```python
from build123d import *

# Parameters (mm, degrees)
CROQUIS1_R              = 1
SALIENTE_EXTRUIR1_DEPTH = 4
CROQUIS1_3_R            = 7
CROQUIS1_3_R_2          = 4
SALIENTE_EXTRUIR2_DEPTH = 6
CHAFL_N1_SIZE           = 3
CHAFL_N2_SIZE           = 3
CHAFL_N2_SIZE_2         = 0.803847577
SALIENTE_EXTRUIR3_DEPTH = 4
MATRIZC1_COUNT          = 36


with BuildPart() as part:
    # Croquis1 → Saliente-Extruir1 (new body)
    with BuildSketch(Plane(origin=(0, 0, 0), x_dir=(1, 0, 0), z_dir=(0, 1, 0))):
        with BuildLine():
            ThreePointArc((-7.395099729, 1.25), (0, -7.5), (7.395099729, 1.25))
            Line((7.395099729, 1.25), (2.958039892, 27.5))
            ThreePointArc((2.958039892, 27.5), (0, 30), (-2.958039892, 27.5))
            Line((-2.958039892, 27.5), (-7.395099729, 1.25))
        make_face()
        with Locations(Location((0, 24, 0), (0, 0, 270))):
            Circle(CROQUIS1_R, mode=Mode.SUBTRACT)
        with Locations(Location((0, 15, 0), (0, 0, 270))):
            Circle(CROQUIS1_R, mode=Mode.SUBTRACT)
        with Locations(Location((0, 18, 0), (0, 0, 270))):
            Circle(CROQUIS1_R, mode=Mode.SUBTRACT)
        with Locations(Location((0, 21, 0), (0, 0, 270))):
            Circle(CROQUIS1_R, mode=Mode.SUBTRACT)
        with Locations(Location((0, 27, 0), (0, 0, 270))):
            Circle(CROQUIS1_R, mode=Mode.SUBTRACT)
        with BuildLine():
            ThreePointArc((-2.988584094, 0.261467228), (-2.974334584, 0.391578577), (-2.954423259, 0.520944533))
            ThreePointArc((-2.954423259, 0.520944533), (2.974334584, -0.391578577), (-2.988584094, 0.261467228))
        make_face(mode=Mode.SUBTRACT)
    extrude(amount=SALIENTE_EXTRUIR1_DEPTH)

    # Croquis1<3> → Saliente-Extruir2 (add)
    # profile 1 of 3: a face of its own
    with BuildSketch(Plane(origin=(0, 0, 0), x_dir=(1, 0, 0), z_dir=(0, 1, 0))):
        with BuildLine():
            ThreePointArc((6.453329346, 3.82158872), (0, 7.5), (-6.453329346, 3.82158872))
            Line((-6.453329346, 3.82158872), (-6.90209308, 1.166666667))
            ThreePointArc((-6.90209308, 1.166666667), (0, 7), (6.90209308, 1.166666667))
            Line((6.90209308, 1.166666667), (6.453329346, 3.82158872))
        make_face()
    # profile 2 of 3: a face of its own
    with BuildSketch(Plane(origin=(0, 0, 0), x_dir=(1, 0, 0), z_dir=(0, 1, 0))):
        with BuildLine():
            Line((-5.662533507, 8.5), (-6.453329346, 3.82158872))
            ThreePointArc((-6.453329346, 3.82158872), (0, 7.5), (6.453329346, 3.82158872))
            Line((6.453329346, 3.82158872), (5.662533507, 8.5))
            Line((5.662533507, 8.5), (-5.662533507, 8.5))
        make_face()
    # profile 3 of 3: a face of its own
    with BuildSketch(Plane(origin=(0, 0, 0), x_dir=(1, 0, 0), z_dir=(0, 1, 0))):
        Circle(CROQUIS1_3_R)
        with Locations(Location((0, 0, 0), (0, 0, 270))):
            Circle(CROQUIS1_3_R_2, mode=Mode.SUBTRACT)
    extrude(amount=SALIENTE_EXTRUIR2_DEPTH)

    # Chaflán1
    # the kernel refuses this chamfer: 3 mm, written as the material it adds along each edge
    with BuildSketch(Plane(origin=(-13.377582471, 4, -8.5), x_dir=(0, -0.02749587661058635, -0.9996219169112968), z_dir=(1, 0, 0))) as chafl_n1_piece_1_section:
        Polygon((CHAFL_N1_SIZE * 0.999621916911, CHAFL_N1_SIZE * 0.0274958766106), (-CHAFL_N1_SIZE * 0.0274958766106, CHAFL_N1_SIZE * 0.999621916911), (0, 0), align=None)
    chafl_n1_piece_1 = extrude(amount=26.755164941, mode=Mode.PRIVATE)
    chafl_n1_piece_1 = split(chafl_n1_piece_1, bisect_by=Plane(origin=(5.328597363, 4.798690402, -10.475592868), z_dir=(-0.9860132971832695, 0, 0.16666666666666669)), keep=Keep.TOP, mode=Mode.PRIVATE)
    chafl_n1_piece_1 = split(chafl_n1_piece_1, bisect_by=Plane(origin=(-5.328597363, 4.798690402, -10.475592868), z_dir=(0.9860132971832695, 0, 0.16666666666666669)), keep=Keep.TOP, mode=Mode.PRIVATE)
    chafl_n1_piece_1 = split(chafl_n1_piece_1, bisect_by=Plane(origin=(0, 6, -9.574895522), z_dir=(0, -1, 0)), keep=Keep.TOP, mode=Mode.PRIVATE)
    add(chafl_n1_piece_1)

    # Chaflán2
    # the kernel refuses this chamfer: 3, 0.803847577 mm, written as the material it takes off along each edge
    with BuildSketch(Plane(origin=(6.90209308, 6, -1.166666667), x_dir=(0.00982773906125155, -0.9999503267608272, -0.0016611910963950731), z_dir=(-0.1666666666666078, 0, -0.9860132971832793))) as chafl_n2_piece_1_section:
        Polygon((CHAFL_N2_SIZE * 0.999950326761, CHAFL_N2_SIZE * 0.00996714657715), (-CHAFL_N2_SIZE_2 * 0.00996714658201, CHAFL_N2_SIZE_2 * 0.999950327126), (0, 0), align=None)
    chafl_n2_piece_1 = extrude(amount=16.241707258, mode=Mode.PRIVATE)
    chafl_n2_piece_1 = split(chafl_n2_piece_1, bisect_by=Plane(origin=(5.281191702, 4, -9.128733123), z_dir=(0, 1, 0)), keep=Keep.TOP, mode=Mode.PRIVATE)
    add(chafl_n2_piece_1, mode=Mode.SUBTRACT)
    with BuildSketch(Plane(origin=(-6.90209308, 6, -1.166666667), x_dir=(0.976646209142954, 0.13751244702122697, 0.16508333980426884), z_dir=(0.1666666666666078, 0, -0.9860132971832793))) as chafl_n2_piece_2_section:
        Polygon((CHAFL_N2_SIZE_2 * 0.990500039187, CHAFL_N2_SIZE_2 * 0.137512447071), (-CHAFL_N2_SIZE * 0.137512447022, CHAFL_N2_SIZE * 0.990500038826), (0, 0), align=None)
    chafl_n2_piece_2 = extrude(amount=16.241707258, mode=Mode.PRIVATE)
    chafl_n2_piece_2 = split(chafl_n2_piece_2, bisect_by=Plane(origin=(-5.281191702, 4, -9.128733123), z_dir=(0, 1, 0)), keep=Keep.TOP, mode=Mode.PRIVATE)
    add(chafl_n2_piece_2, mode=Mode.SUBTRACT)
    with BuildSketch(Plane(origin=(0, 6, 0), x_dir=(0.9860132971832691, 0, -0.16666666666666757), z_dir=(-0.16666666666666757, 0, -0.9860132971832691))) as chafl_n2_piece_3_section:
        Polygon((7, CHAFL_N2_SIZE), (7 - CHAFL_N2_SIZE_2, 0), (7, 0), align=None)
    chafl_n2_piece_3 = revolve(axis=Axis((0, 6, 0), (0, -1, 0)), revolution_arc=199.188136454, mode=Mode.PRIVATE)
    chafl_n2_piece_3 = split(chafl_n2_piece_3, bisect_by=Plane(origin=(0, 4, 6.478370391), z_dir=(0, 1, 0)), keep=Keep.TOP, mode=Mode.PRIVATE)
    add(chafl_n2_piece_3, mode=Mode.SUBTRACT)

    # Croquis1<4> → Saliente-Extruir3 (add)
    with BuildSketch(Plane(origin=(0, 0, 0), x_dir=(1, 0, 0), z_dir=(0, 1, 0))):
        with BuildLine():
            Line((-3, 0), (-2.73953542, 0.239678293))
            Line((-2.73953542, 0.239678293), (-2.988584094, 0.261467228))
            ThreePointArc((-2.988584094, 0.261467228), (-2.997144665, 0.130858162), (-3, 0))
        make_face()
        with BuildLine():
            Line((-2.988584094, 0.261467228), (-2.73953542, 0.239678293))
            Line((-2.73953542, 0.239678293), (-2.954423259, 0.520944533))
            ThreePointArc((-2.954423259, 0.520944533), (-2.974334584, 0.391578577), (-2.988584094, 0.261467228))
        make_face()
    saliente_extruir3 = extrude(amount=SALIENTE_EXTRUIR3_DEPTH)

    # MatrizC1: Saliente-Extruir3 ×36 about axis
    matrizc1_axis = Axis((0, 0, 0), (0, 1, 0))
    for i in range(1, MATRIZC1_COUNT):
        add(saliente_extruir3.rotate(matrizc1_axis, i * 360 / MATRIZC1_COUNT))


solid = part.part
```
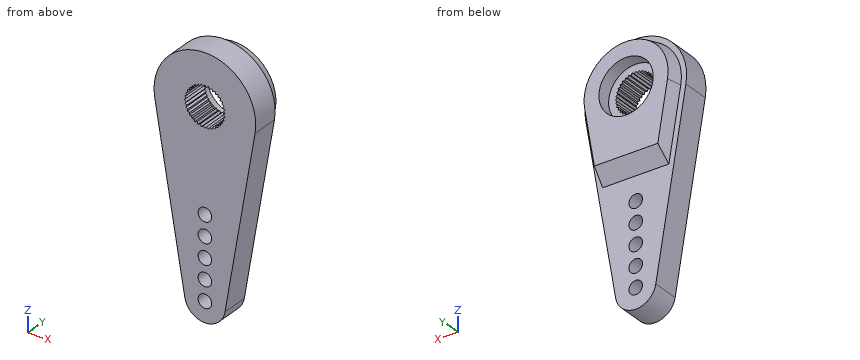
Geometry: final body of the model. Coordinates: model frame, mm. Round coordinates to 2 decimals unless told otherwise and drop trailing zeros. Write each loop counter-clockwise with the first axis right and the second up, starting at its lowest first coordinate (ties: lowest second). Pieces come first, ordered by that corner, then holes. Notation, with made-up numbers: (39.5, 51) -> (91.5, 51) arc R14 ccw to (91.5, 76) -> close; hole circle Ø11 at (81.5, 11). An arc over 180 degrees is marked (long way). Use CSV: the item, a comma, the result in double quotes. Start each with the question number.
Q1. Section D-D (z = -18). Return loops of the section in (x, y), plus the area to 3 significant figures.
Q2. First-contact query: pin 1 Ø1.8 at (x, z) = (0, -24) entering from -Y. Flat tip, straight axial feed; report the tip coordinate or a pass-through.
Q3. Line query: L1, parallel to X at y = 4.5, z = -3.5; L2, parallel to X at y = 2.5, z = -18.5; L3, parallel to X at y = 2.5, z = -7. Output: solid intervals per line, ascending.
Q4. Section C-C (y = 1.25). Give the number of separate pieces and of enclosed holes in the cut face, plus the area to 3 significant figures.
Q5. Section B-B (z = -7). Return loops of the section in (x, y), plus the area to 3 significant figures.
Q6. Section A-A (z = -24). Return loops of the section in (x, y).
Result sheet:
1,outline,"(-4.56, 0) -> (-1, 0) -> (-1, 4) -> (-4.56, 4) -> close; (1, 0) -> (4.56, 0) -> (4.56, 4) -> (1, 4) -> close"
1,area,"28.5 mm²"
2,pin 1,"through"
3,L1,"-6.1 to -1.94, 1.94 to 6.1"
3,L2,"-4.48 to -0.87, 0.87 to 4.48"
3,L3,"-6.42 to 6.42"
4,separate pieces,"1"
4,enclosed holes,"6"
4,area,"348 mm²"
5,outline,"(-6.42, 0) -> (6.42, 0) -> (6.42, 4) -> (5.64, 4) -> (5.1, 6) -> (-5.1, 6) -> (-5.64, 4) -> (-6.42, 4) -> close"
5,area,"72.9 mm²"
6,outline,"(-3.55, 0) -> (-1, 0) -> (-1, 4) -> (-3.55, 4) -> close; (1, 0) -> (3.55, 0) -> (3.55, 4) -> (1, 4) -> close"
